Answer from the drawing. Dimensions are ordinates in mm from the lowest x, y and z of the part. A direction names the side the tool comes from. Round coordinates to 2 decimals unless told otherwise and drop trailing zeros. Write each loop counter-clockwise with the first axis right and the second up, starting at its lowest first coordinate (ties: lowest second). Pieces come first, ordered by that corner, then holes. Notation, with made-up numbers: (-38.5, -35) - (-7.5, -35) arc R29 cw to (-7.5, -4) - close; hole circle Ø1 at (-5.75, 65.5). An arc over 180 degrees is marked (long way). Answer as CSV lines item,"result". Start each with the question number.
1) Find section D-D on y = 14. Determine the outline of the cut face in (x, z), then the cut area to 3 significant figures.
2) For a pull along X with two mould halves and no side action, classify the marked faces 4, 5, 6 and 7 as +X half, -X half, draft (parallel to the pull), parting line (faces both ways), or undercut.
3) Consider line 1 along X through (y, z) = (32, 15); line 2 along Y through (x, z) = (16, 40); line 3 along Z through (x, y) = (32, 14.5). Determine where each line is inside the solid, lowest interval first.
4) Find section C-C on x = 14. Determine the outline of the cut face in (y, z).
5) Each of these flat-tipped pins is pushed along its axis until it touches: pin 1 (4 mm diameter, centred on x = 23, z = 79, fed in from +Y); pin 2 (3.5 mm diameter, centred on x = 19.5, z = 20.5, fed in from +Y); pin 3 (12 mm diameter, centred on x = 13, y = 29.5, fed in from -Z). Where does it stop, or does it pass through?
6) Find section B-B on y = 34. Determine the outline of the cut face in (x, z).
7) Which of the six approach directions +Z, -Z, +X, -X, +Y, -Y give full straight-line access (tool end or side, diameter ignored) to the marked faces 1, 2 and 3?
8) Find section A-A on z = 70. Determine the outline of the cut face in (x, y), then the cut area to 3 significant figures.
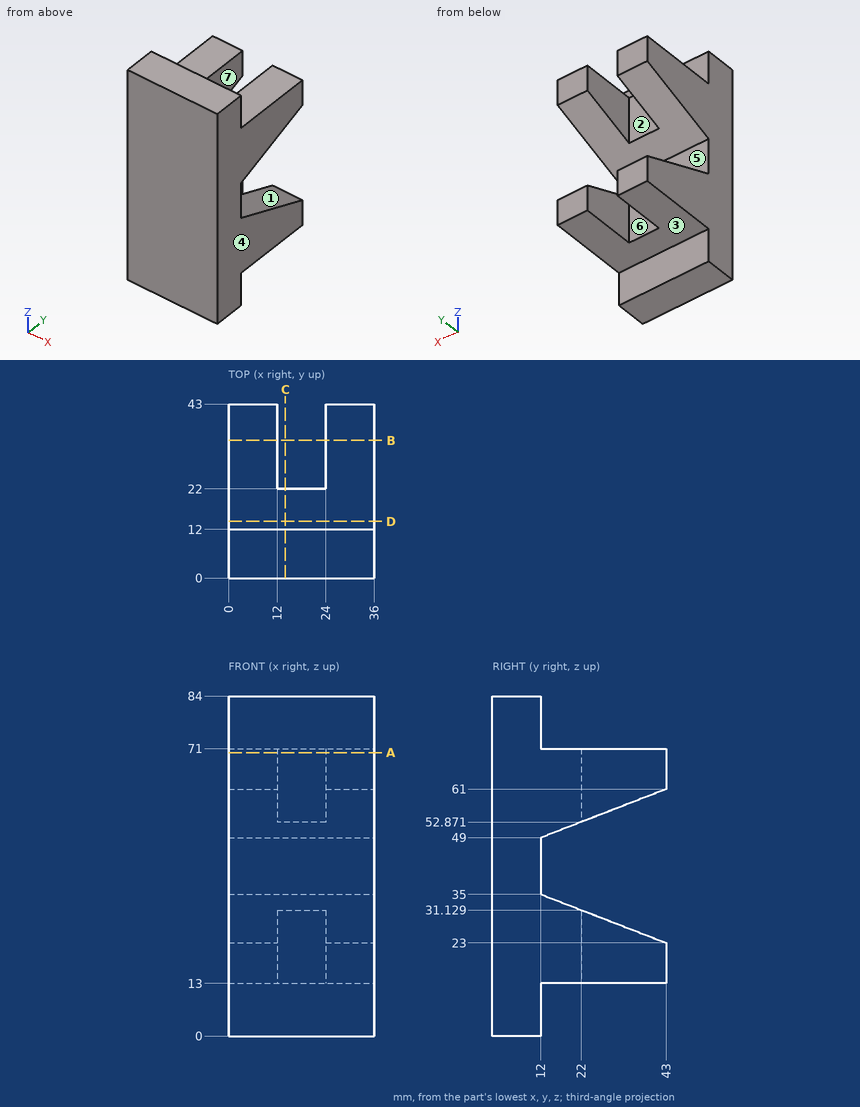
Check values:
1,outline,"(0, 13) - (36, 13) - (36, 34.23) - (0, 34.23) - close; (0, 49.77) - (36, 49.77) - (36, 71) - (0, 71) - close"
1,area,"1,530 mm^2"
2,face 4,"+X half"
2,face 5,"draft"
2,face 6,"undercut"
2,face 7,"undercut"
3,line 1,"x = 0 to 12, 24 to 36"
3,line 2,"y = 0 to 12"
3,line 3,"z = 13 to 34.03, 49.97 to 71"
4,outline,"(0, 0) - (12, 0) - (12, 13) - (22, 13) - (22, 31.13) - (12, 35) - (12, 49) - (22, 52.87) - (22, 71) - (12, 71) - (12, 84) - (0, 84) - close"
5,pin 1,"stops at y = 12"
5,pin 2,"stops at y = 22"
5,pin 3,"stops at z = 13"
6,outline,"(0, 13) - (12, 13) - (12, 26.48) - (0, 26.48) - close; (0, 57.52) - (12, 57.52) - (12, 71) - (0, 71) - close; (24, 13) - (36, 13) - (36, 26.48) - (24, 26.48) - close; (24, 57.52) - (36, 57.52) - (36, 71) - (24, 71) - close"
7,face 1,"+X, -X, +Y"
7,face 2,"+Z, -Z, +Y"
7,face 3,"-Z, +X, -X, +Y"
8,outline,"(0, 0) - (36, 0) - (36, 43) - (24, 43) - (24, 22) - (12, 22) - (12, 43) - (0, 43) - close"
8,area,"1,300 mm^2"
